Input: part model. Units: mm. Frame: model coordinates. Face numbers are marked on the shaded views. A direction names the side the tool comes from. Coordinates: 2 decimals unless noted, no trailing zeros. Order: outer loops, then holes, each group sorted by start corner. A loop starts at its lowest first (then second) coordinate and runs counter-clockwise, first axis right, second up. Notation, with made-up numbers: (-14, 71) -> (17, 71) arc R20 cw to (17, 92) -> close; hole circle Ø10 at (-36.75, 34.25). An arc over 180 degrees is marked (long way). Use one line per item in the form item = value. Start each with the question number.
1) Pin query (flat end, axial travel): pin 1 (5 mm diameter, centred on x = -1.5, y = 3.5, fed in from -Z); pin 2 (2.5 mm diameter, centred on x = 1, y = -7, fed in from +Z). Return the tip coordinate at first contact, or that it passes through.
2) Access query for the marked faces 4, 5 and 6. Directions: +Z, -Z, +X, -X, +Y, -Y. A direction counts if a zero-diameter tool reaches every point of the face in a straight line with its end or side. Return the directions, or none.
3) Draft query along Y for the marked faces 1, 2 and 3. Return one class per face: pulls with the +Y half, pulls with the -Y half, needs draft (parallel to the pull), parting line crosses it, or undercut.
4) Section query C-C on z = -0.5. Output: boundary loops of the cut face in (x, y), then the cut area to 3 significant figures.
5) Section query A-A on y = 4.5. Output: boundary loops of the cut face in (x, z).
6) Section query D-D on y = 1.25. Output: boundary loops of the cut face in (x, z), then the cut area to 3 significant figures.
7) Section query B-B on x = 17. Output: boundary loops of the cut face in (y, z), then the cut area to 3 significant figures.
8) Ray query, line 1 along X through (y, z) = (8.5, -2.5); line 2 along Y through (x, z) = (-12.5, -6.25); line 3 along X through (y, z) = (-0.75, -2.5). Return the intervals inside material, ascending.
from build123d import *

# Parameters (mm, degrees)
BOSS_EXTRUDE1_DEPTH = 8
SKETCH2_W           = 23
SKETCH2_H           = 3
CUT_EXTRUDE1_DEPTH  = 4
FILLET1_R           = 1
FILLET2_R           = 1


with BuildPart() as part:
    # Sketch1 → Boss-Extrude1 (new body)
    with BuildSketch(Plane.XY):
        with BuildLine():
            ThreePointArc((15.076086957, 0.60326087), (16.576086957, 2.10326087), (18.076086957, 0.60326087))
            Line((18.076086957, 0.60326087), (24.076086957, 0.60326087))
            Line((24.076086957, 0.60326087), (24.076086957, 6.60326087))
            Line((24.076086957, 6.60326087), (24.076086957, 9.60326087))
            Line((24.076086957, 9.60326087), (13.076086957, 9.60326087))
            Line((13.076086957, 9.60326087), (-9.923913043, 9.60326087))
            Line((-9.923913043, 9.60326087), (-15.923913043, 9.60326087))
            Line((-15.923913043, 9.60326087), (-15.923913043, 6.60326087))
            Line((-15.923913043, 6.60326087), (-15.923913043, 0.60326087))
            Line((-15.923913043, 0.60326087), (-13.923913043, 0.60326087))
            ThreePointArc((-13.923913043, 0.60326087), (-12.423913043, 2.10326087), (-10.923913043, 0.60326087))
            Line((-10.923913043, 0.60326087), (-9.923913043, 0.60326087))
            Line((-9.923913043, 0.60326087), (-9.923913043, 6.60326087))
            Line((-9.923913043, 6.60326087), (13.076086957, 6.60326087))
            Line((13.076086957, 6.60326087), (13.076086957, 0.60326087))
            Line((13.076086957, 0.60326087), (15.076086957, 0.60326087))
        make_face()
        with BuildLine():
            Line((24.076086957, 0.60326087), (18.076086957, 0.60326087))
            ThreePointArc((18.076086957, 0.60326087), (16.576086957, -0.89673913), (15.076086957, 0.60326087))
            Line((15.076086957, 0.60326087), (13.076086957, 0.60326087))
            Line((13.076086957, 0.60326087), (13.076086957, -5.39673913))
            Line((13.076086957, -5.39673913), (-9.923913043, -5.39673913))
            Line((-9.923913043, -5.39673913), (-9.923913043, 0.60326087))
            Line((-9.923913043, 0.60326087), (-10.923913043, 0.60326087))
            ThreePointArc((-10.923913043, 0.60326087), (-12.423913043, -0.89673913), (-13.923913043, 0.60326087))
            Line((-13.923913043, 0.60326087), (-15.923913043, 0.60326087))
            Line((-15.923913043, 0.60326087), (-15.923913043, -5.39673913))
            Line((-15.923913043, -5.39673913), (-15.923913043, -8.39673913))
            Line((-15.923913043, -8.39673913), (-9.923913043, -8.39673913))
            Line((-9.923913043, -8.39673913), (13.076086957, -8.39673913))
            Line((13.076086957, -8.39673913), (24.076086957, -8.39673913))
            Line((24.076086957, -8.39673913), (24.076086957, -5.39673913))
            Line((24.076086957, -5.39673913), (24.076086957, 0.60326087))
        make_face()
    extrude(amount=-BOSS_EXTRUDE1_DEPTH)

    # Sketch2 → Cut-Extrude1 (cut)
    with BuildSketch(Plane.XY):
        with Locations((1.576086957, 8.10326087)):
            Rectangle(SKETCH2_W, SKETCH2_H)
        with Locations((1.576086957, -6.89673913)):
            Rectangle(SKETCH2_W, SKETCH2_H)
    extrude(amount=-CUT_EXTRUDE1_DEPTH, mode=Mode.SUBTRACT)

    # Fillet1
    fillet1_edges = [part.edges().sort_by_distance(p)[0] for p in [
        (-9.923913043, 8.10326087, -4),
        (13.076086957, 8.10326087, -4),
        (-9.923913043, -6.89673913, -4),
        (13.076086957, -6.89673913, -4),
    ]]
    fillet(fillet1_edges, radius=FILLET1_R)

    # Fillet2
    fillet2_edges = [part.edges().sort_by_distance(p)[0] for p in [
        (-15.923913043, 9.60326087, -4),
        (24.076086957, 9.60326087, -4),
    ]]
    fillet(fillet2_edges, radius=FILLET2_R)


solid = part.part
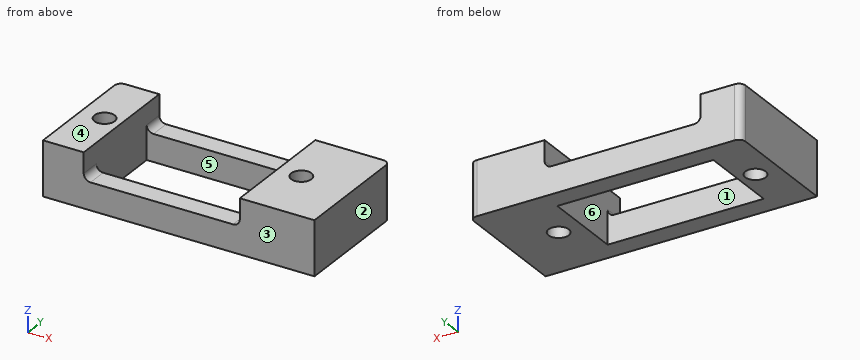
Answers below:
q1.pin_1 = through
q1.pin_2 = -4
q2.face_4 = +Z, +X, -X, +Y, -Y
q2.face_5 = +Z, -Z
q2.face_6 = +Z
q3.face_1 = undercut
q3.face_2 = needs draft
q3.face_3 = pulls with the -Y half
q4.outline = (-15.92, -8.4) -> (-9.92, -8.4) -> (-9.92, 9.6) -> (-14.92, 9.6) arc R1 ccw to (-15.92, 8.6) -> close; (13.08, -8.4) -> (24.08, -8.4) -> (24.08, 8.6) arc R1 ccw to (23.08, 9.6) -> (13.08, 9.6) -> close; hole circle Ø3 at (-12.42, 0.6); hole circle Ø3 at (16.58, 0.6)
q4.area = 291 mm^2
q5.outline = (-15.92, -8) -> (-9.92, -8) -> (-9.92, 0) -> (-15.92, 0) -> close; (13.08, -8) -> (24.08, -8) -> (24.08, 0) -> (13.08, 0) -> close
q6.outline = (-15.92, -8) -> (-13.78, -8) -> (-13.78, 0) -> (-15.92, 0) -> close; (-11.07, -8) -> (-9.92, -8) -> (-9.92, 0) -> (-11.07, 0) -> close; (13.08, -8) -> (15.22, -8) -> (15.22, 0) -> (13.08, 0) -> close; (17.93, -8) -> (24.08, -8) -> (24.08, 0) -> (17.93, 0) -> close
q6.area = 92.7 mm^2
q7.outline = (-8.4, -8) -> (-0.84, -8) -> (-0.84, 0) -> (-8.4, 0) -> close; (2.04, -8) -> (9.6, -8) -> (9.6, 0) -> (2.04, 0) -> close
q7.area = 121 mm^2
q8.line_1 = -15.92 to -9.92, 13.08 to 24.08
q8.line_2 = -8.4 to -0.89, 2.1 to 9.6
q8.line_3 = -15.92 to -13.07, -11.78 to -9.92, 13.08 to 15.93, 17.22 to 24.08
